Here's how the part is built. I have some questions about the finished solid (model axes, mm). Round coordinates to 2 decimals unless told otherwise and drop trailing zeros. Use a Markdown table: item, result.
```python
from build123d import *

# Parameters (mm, degrees)
SKETCH_1_W          = 70
SKETCH_1_H          = 130
EXTRUDE_1_DEPTH     = 4
SKETCH_2_R          = 2
CUT_EXTRUDE_1_DEPTH = 10
FILLET_1_R          = 6
CHAMFER_1_SIZE      = 2
SKETCH_3_R          = 2
CUT_EXTRUDE_2_DEPTH = 15
CHAMFER_2_SIZE      = 1.9
SKETCH_4_R          = 2.5
CUT_EXTRUDE_3_DEPTH = 15
CHAMFER_3_SIZE      = 2.9
SKETCH_5_R          = 1.5
CUT_EXTRUDE_4_DEPTH = 12


with BuildPart() as part:
    # Эскиз1 → Бобышка-Вытянуть1 (new body)
    with BuildSketch(Plane(origin=(0, 0, 0), x_dir=(0, 0, -1), z_dir=(1, 0, 0))):
        with Locations((15.001853179, -3.931833533)):
            Rectangle(SKETCH_1_W, SKETCH_1_H)
    extrude(amount=EXTRUDE_1_DEPTH)

    # Эскиз2 → Вырез-Вытянуть1 (cut)
    with BuildSketch(Plane.ZY):
        with Locations((-28.001653179, -28.231733533)):
            Circle(SKETCH_2_R)
        with Locations((-28.001653179, -54.231733533)):
            Circle(SKETCH_2_R)
        with Locations((-2.001653179, -28.231733533)):
            Circle(SKETCH_2_R)
        with Locations((-2.001653179, -54.231733533)):
            Circle(SKETCH_2_R)
    extrude(amount=-CUT_EXTRUDE_1_DEPTH, mode=Mode.SUBTRACT)

    # Скругление1
    fillet_1_edges = [part.edges().sort_by_distance(p)[0] for p in [
        (2, 61.068166467, 19.998146821),
        (2, 61.068166467, -50.001853179),
        (2, -68.931833533, -50.001853179),
        (2, -68.931833533, 19.998146821),
    ]]
    fillet(fillet_1_edges, radius=FILLET_1_R)

    # Фаска1
    chamfer_1_edges = [part.edges().sort_by_distance(p)[0] for p in [
        (0, -28.231733533, -30.001653179),
        (0, -54.231733533, -30.001653179),
        (0, -28.231733533, -4.001653179),
        (0, -54.231733533, -4.001653179),
    ]]
    chamfer(chamfer_1_edges, length=CHAMFER_1_SIZE)

    # Эскиз3 → Вырез-Вытянуть2 (cut)
    with BuildSketch(Plane.ZY):
        with Locations((13.998146821, 55.068166467)):
            Circle(SKETCH_3_R)
        with Locations((13.998146821, -62.931833533)):
            Circle(SKETCH_3_R)
        with Locations((13.998146821, -3.931833533)):
            Circle(SKETCH_3_R)
    extrude(amount=-CUT_EXTRUDE_2_DEPTH, mode=Mode.SUBTRACT)

    # Фаска2
    chamfer_2_edges = [part.edges().sort_by_distance(p)[0] for p in [
        (0, 55.068166467, 11.998146821),
        (0, -62.931833533, 11.998146821),
        (0, -3.931833533, 11.998146821),
    ]]
    chamfer(chamfer_2_edges, length=CHAMFER_2_SIZE)

    # Эскиз4 → Вырез-Вытянуть3 (cut)
    with BuildSketch(Plane(origin=(4, 0, 0), x_dir=(0, 0, -1), z_dir=(1, 0, 0))):
        with Locations((-7.998146821, -15.531833533)):
            Circle(SKETCH_4_R)
        with Locations((38.001853179, -15.531833533)):
            Circle(SKETCH_4_R)
    extrude(amount=-CUT_EXTRUDE_3_DEPTH, mode=Mode.SUBTRACT)

    # Фаска3
    chamfer_3_edges = [part.edges().sort_by_distance(p)[0] for p in [
        (4, -15.531833533, -35.501853179),
        (4, -15.531833533, 10.498146821),
    ]]
    chamfer(chamfer_3_edges, length=CHAMFER_3_SIZE)

    # Эскиз5 → Вырез-Вытянуть4 (cut)
    with BuildSketch(Plane.ZY):
        with Locations((-15.001853179, 4.068166467)):
            Circle(SKETCH_5_R)
    extrude(amount=-CUT_EXTRUDE_4_DEPTH, mode=Mode.SUBTRACT)


solid = part.part
```
Q1. I need wall thicknesses on line 1 (Y direction, x = 1.05, z = -28.5); line 2 (Z direction, x = 1.6, y = -29); line 3 (Y direction, x = 0.45, z = 14). Which ranges of each line are inside material? Lowest first, please. Write a range as from..to.
Return value:
| item | result |
|---|---|
| line 1 | y = -68.93..-57.14, -51.32..-31.14, -25.32..61.07 |
| line 2 | z = -50..-30.28, -25.73..-4.28, 0.27..20 |
| line 3 | y = -68.93..-66.38, -59.48..-7.38, -0.48..51.62, 58.52..61.07 |
Q2. Imagine slicing it at A-A, the plane x = 3.3. Give the number of separate pieces and of enclosed holes in the cut face, then the cut area to 3 significant figures.
Return value:
| item | result |
|---|---|
| separate pieces | 1 |
| enclosed holes | 10 |
| area | 8,840 mm^2 |
Q3. We'd pull the mould along Z, two halves only. Please class faces 1 (the cylindrical face through (0.56, -16.49, -40.31)), 2 (the flat face through (2, -5, -50.002)), 3 (the flat face through (4, -3, -15)): pulls with the +Z half, pulls with the -Z half, needs draft (parallel to the pull), parting line crosses it, or undercut.
Return value:
| item | result |
|---|---|
| face 1 | undercut |
| face 2 | pulls with the -Z half |
| face 3 | needs draft |
Q4. Will these pins go through, and if not, where does the flat tip stop? P1, Ø6.5, axis at y = -28.23, z = -2, coming from the -X side; P2, Ø4, axis at y = 4.07, z = -15, coming from the +X side; P3, Ø4.5, axis at y = -54.23, z = -28, coming from the -X side; P4, Ø8, axis at y = -15.53, z = 8, coming from the +X side.
Return value:
| item | result |
|---|---|
| P1 | stops at x = 0.75 |
| P2 | stops at x = 4 |
| P3 | stops at x = 1.75 |
| P4 | stops at x = 2.6 |
